```python
from build123d import *

# Parameters (mm, degrees)
SKETCH1_W           = 89
SKETCH1_H           = 29
SKETCH1_W_2         = 77
SKETCH1_H_2         = 17
BOSS_EXTRUDE1_DEPTH = 5
FILLET1_R           = 4
DRAFT1_ANGLE        = 4


with BuildPart() as part:
    # Sketch1 → Boss-Extrude1 (new body)
    with BuildSketch(Plane.XY):
        Rectangle(SKETCH1_W, SKETCH1_H)
        Rectangle(SKETCH1_W_2, SKETCH1_H_2, mode=Mode.SUBTRACT)
    extrude(amount=BOSS_EXTRUDE1_DEPTH)

    # Fillet1
    fillet1_edges = [part.edges().sort_by_distance(p)[0] for p in [
        (44.5, -14.5, 2.5),
        (-44.5, -14.5, 2.5),
        (-44.5, 14.5, 2.5),
        (44.5, 14.5, 2.5),
    ]]
    fillet(fillet1_edges, radius=FILLET1_R)

    # Draft1
    draft1_faces = [part.faces().sort_by_distance(p)[0] for p in [
        (38.5, 0, 2.5),
        (0, -8.5, 2.5),
        (-38.5, 0, 2.5),
        (0, 8.5, 2.5),
    ]]
    draft(draft1_faces, Plane.XY.offset(5), DRAFT1_ANGLE)


solid = part.part
```
Verification items for the finished model (mm, model axes). A direction names the side the tool comes from. Round coordinates to 2 decimals unless told otherwise and drop trailing zeros. Order: outer loops, then holes, each group sorted by start corner. A loop starts at its lowest first (then second) coordinate and runs counter-clockwise, first axis right, second up. Notation, with made-up numbers: (16, 28) -> (61, 28) arc R23 cw to (61, 57) -> close; hole circle Ø7 at (40, 84.5). An arc over 180 degrees is marked (long way). Put each result on its own line as item: value. Start each with the question number.
(1) Tool access check on faces 4 (the face through (-0.539, -8.323, 2.465)), 5 (the face through (-44.5, 0, 2)). Record the directions out of +Z, -Z, +X, -X, +Y, -Y that give a thin tool (end or side, any length) a straight path to the whole face; none if there is none.
(2) Depth check by flat-ended pin: pin 1 Ø1 at (y, z) = (-11.5, 2) entering from -X. Enter the tip coordinate at first touch or a pass-through.
(3) Material ranges on line 1 along X through (y, z) = (-6.25, 0.25); line 2 along X through (y, z) = (-6, 4.05); line 3 along Y through (x, z) = (19, 1.35), recorded low to high.
(4) Section check A-A (x = -3). Enter the section's corners in (y, z).
(5) Section check C-C (z = 2.9). Enter the section's corners in (x, y), then the cut area to 3 significant figures.
(6) Section check B-B (y = -6.25). Enter the section's corners in (x, z).
(7) Draft check along X on faces 1 (the face through (-43.359, -13.297, 2.535)), 2 (the face through (38.323, -0.119, 2.465)), 3 (the face through (-1, 10, 0)). Enter one of: +X half, -X half, draft (parallel to the pull), parting line (faces both ways), or undercut.
Completed:
1. face 4: +Z
1. face 5: +Z, -Z, -X, +Y, -Y
2. pin 1: stops at x = -44.47
3. line 1: x = -44.5 to -38.17, 38.17 to 44.5
3. line 2: x = -44.5 to -38.43, 38.43 to 44.5
3. line 3: y = -14.5 to -8.24, 8.24 to 14.5
4. outline: (-14.5, 0) -> (-8.15, 0) -> (-8.5, 5) -> (-14.5, 5) -> close; (8.15, 0) -> (14.5, 0) -> (14.5, 5) -> (8.5, 5) -> close
5. outline: (-44.5, -10.5) arc R4 ccw to (-40.5, -14.5) -> (40.5, -14.5) arc R4 ccw to (44.5, -10.5) -> (44.5, 10.5) arc R4 ccw to (40.5, 14.5) -> (-40.5, 14.5) arc R4 ccw to (-44.5, 10.5) -> close; hole (-38.35, -8.35) -> (38.35, -8.35) -> (38.35, 8.35) -> (-38.35, 8.35) -> close
5. area: 1,290 mm2
6. outline: (-44.5, 0) -> (-38.15, 0) -> (-38.5, 5) -> (-44.5, 5) -> close; (38.15, 0) -> (44.5, 0) -> (44.5, 5) -> (38.5, 5) -> close
7. face 1: -X half
7. face 2: undercut
7. face 3: draft
